Build history of the part. All positions in model axes, mm. Face numbers are marked on the shaded views. A direction names the side the tool comes from. Give positions to 0.01 mm unless a question says otherwise; leave off trailing zeros. Order: outer loops, then holes, each group sorted by start corner. A loop starts at its lowest first (then second) coordinate and runs counter-clockwise, first axis right, second up. Notation, with made-up numbers: M -23.5,-9.75 L -18.5,-9.75 A18 ccw -18.5,-5.75 Z; hole C 85.25,12.25 d6. An arc over 180 degrees is marked long. One line per item, written item: value.
from build123d import *

# Parameters (mm, degrees)
PAD003_DEPTH    = 7.5
SKETCH037_W     = 13.73571
SKETCH037_H     = 11.046402
SKETCH037_R     = 1.375
POCKET020_DEPTH = 8
FILLET001_R     = 0.5


with BuildPart() as part:
    # Sketch036 (on DatumPlane) → Pad003 (new body)
    with BuildSketch(Plane.XZ.offset(11)):
        with BuildLine():
            ThreePointArc((-2.977124, 6), (-4.362654, 6.499018), (-5.714214, 5.914214))
            Line((-6.067767, 6.267767), (-5.714214, 5.914214))
            ThreePointArc((-2.646405, 6.375), (-4.378317, 6.998773), (-6.067767, 6.267767))
            ThreePointArc((-2.646405, 6.375), (-2.492463, 6.282293), (-2.315687, 6.25))
            Line((-2.315687, 6.25), (2.300007, 6.25))
            ThreePointArc((2.300007, 6.25), (2.47678, 6.282294), (2.630719, 6.375))
            ThreePointArc((6.05208, 6.267767), (4.362631, 6.998773), (2.630719, 6.375))
            Line((6.05208, 6.267767), (5.698527, 5.914214))
            ThreePointArc((5.698527, 5.914214), (4.346967, 6.499018), (2.961438, 6))
            ThreePointArc((2.3, 5.75), (2.653553, 5.814586), (2.961438, 6))
            Line((2.3, 5.75), (0, 5.75))
            Line((-2.315687, 5.75), (0, 5.75))
            ThreePointArc((-2.977124, 6), (-2.66924, 5.814586), (-2.315687, 5.75))
        make_face()
    extrude(amount=-PAD003_DEPTH)

    # Sketch037 → Pocket020 (cut)
    with BuildSketch(Plane.XY):
        with Locations((-0.219563, -6.661829)):
            Rectangle(SKETCH037_W, SKETCH037_H)
        with BuildLine():
            ThreePointArc((-4.714286, -9.938587), (0, -11), (4.714286, -9.938587))
            ThreePointArc((4.714286, -9.938587), (4.922577, -9.754094), (5, -9.486833))
            Line((5, -9.486833), (5, -3))
            ThreePointArc((5, -3), (4.853553, -2.646447), (4.5, -2.5))
            Line((4.5, -2.5), (-4.5, -2.5))
            ThreePointArc((-4.5, -2.5), (-4.853553, -2.646447), (-5, -3))
            Line((-5, -3), (-5, -9.486833))
            ThreePointArc((-5, -9.486833), (-4.922577, -9.754094), (-4.714286, -9.938587))
        make_face(mode=Mode.SUBTRACT)
        with Locations((0, -5.5)):
            Circle(SKETCH037_R)
        with Locations((0, -9.2)):
            Circle(SKETCH037_R)
    extrude(amount=POCKET020_DEPTH, mode=Mode.SUBTRACT)

    # Fillet001
    fillet001_edges = [part.edges().sort_by_distance(p)[0] for p in [
        (-5, -3.5, 6.63675),
        (5, -3.5, 6.631466),
    ]]
    fillet(fillet001_edges, radius=FILLET001_R)


solid = part.part
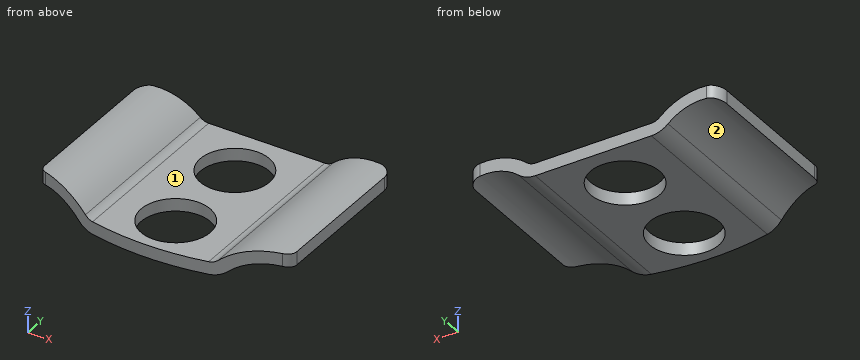
1) Tool access for the marked faces 1 and 2: list every direction of +Z, -Z, +X, -X, +Y, -Y with a clear straight run to the whole face (end or side of a thin tool).
Check values:
face 1: +Z, +Y, -Y
face 2: -Z, +Y, -Y
2) Saw through at A-A, the plane x = 0. Write the cut outline in (y, z) (3 decimals).
Check values:
outline: M -11,5.75 L -10.575,5.75 L -10.575,6.25 L -11,6.25 Z; M -7.825,5.75 L -6.875,5.75 L -6.875,6.25 L -7.825,6.25 Z; M -4.125,5.75 L -3.5,5.75 L -3.5,6.25 L -4.125,6.25 Z
3) Saw through at D-D, the plane x = 1.25. Write the cut outline in (y, z), then the cut area to 3 significant figures.
Check values:
outline: M -10.93,5.75 L -9.77,5.75 L -9.77,6.25 L -10.93,6.25 Z; M -8.63,5.75 L -6.07,5.75 L -6.07,6.25 L -8.63,6.25 Z; M -4.93,5.75 L -3.5,5.75 L -3.5,6.25 L -4.93,6.25 Z
area: 2.57 mm^2
4) Pin check, flat tips, straight feed: pin 1 (3.5 mm diameter, centred on x = 0.5, y = -6.5, fed in from +Z); pin 2 (2 mm diameter, centred on x = 0, y = -9.2, fed in from +Z); pin 3 (4 mm diameter, centred on x = 0.5, y = -7.5, fed in from +Z). Stop position of each tip, or through.
Check values:
pin 1: z = 6.25
pin 2: through
pin 3: z = 6.29
5) Drill centre lines: probe 1 along Y at (x, z) = (0, 6.05) (3 decimals); probe 2 along X at (y, z) = (-5.5, 6) (3 decimals); probe 3 along Z at (x, y) = (2, -8.75). Where is each one in solid material? Low to high. Write a range as from..to.
Check values:
probe 1: -11..-10.575, -7.825..-6.875, -4.125..-3.5
probe 2: -2.977..-1.375, 1.375..2.961
probe 3: 5.75..6.25
